from build123d import *

# Parameters (mm, degrees)
SKETCH_W     = 6
SKETCH_H     = 10
PAD_DEPTH    = 2
SKETCH001_W  = 2
SKETCH001_H  = 10
PAD001_DEPTH = 6.5
CHAMFER_SIZE = 1


with BuildPart() as part:
    # Sketch → Pad (new body)
    with BuildSketch(Plane.XY):
        Rectangle(SKETCH_W, SKETCH_H)
    extrude(amount=PAD_DEPTH)

    # Sketch001 (on Face6 of Pad) → Pad001 (join)
    with BuildSketch(Plane.XY.offset(2)):
        with Locations((-2, 0)):
            Rectangle(SKETCH001_W, SKETCH001_H)
        with Locations((2, 0)):
            Rectangle(SKETCH001_W, SKETCH001_H)
    extrude(amount=PAD001_DEPTH)

    # Chamfer
    chamfer_edges = [part.edges().sort_by_distance(p)[0] for p in [
        (-1, -5, 5.25),
        (1, -5, 5.25),
        (-1, 5, 5.25),
        (1, 5, 5.25),
    ]]
    chamfer(chamfer_edges, length=CHAMFER_SIZE)


solid = part.part
Verification items for the finished model (mm, model axes). A direction names the side the tool comes from. Round coordinates to 2 decimals unless told otherwise and drop trailing zeros. Loops run counter-clockwise (first coordinate to the right, second up) from the corner with the lowest first, then second, coordinate; pieces in that order, holes last. Notation, with made-up numbers: M 25,-26 L 77,-26 A24 ccw 77,-6 Z; hole C 27,78 d2. An arc over 180 degrees is marked long. Write each question's results on one line, items separated by ' | '.
1) Section check A-A on z = 6.5. Record the boundary of the cut face in (x, y), then the cut area to 3 significant figures.
Checks:
outline: M -3,-5 L -2,-5 L -1,-4 L -1,4 L -2,5 L -3,5 Z; M 1,-4 L 2,-5 L 3,-5 L 3,5 L 2,5 L 1,4 Z | area: 38.0 mm2
2) Section check D-D on x = -0.15. Record the boundary of the cut face in (y, z).
Checks:
outline: M -5,0 L 5,0 L 5,2 L -5,2 Z
3) Mould release check, pull along X, two halves, no side actions. Record for faces 1 (the flat face through (-3, 0, 4)), 2 (the flat face through (-2, 0, 8.5)), 3 (the flat face through (1.5, 4.5, 5.2)): released by +X, released by -X, zero draft, split by the parting line, or undercut.
Checks:
face 1: released by -X | face 2: zero draft | face 3: undercut
4) Scan lines: L1, parallel to X at y = 1, z = 6.5; L2, parallel to X at y = -4.5, z = 5.5; L3, parallel to Z at x = 0.6, y = -3.25. Record each from-to range of solid material in increasing order. Write a range as from..to.
Checks:
L1: x = -3..-1, 1..3 | L2: x = -3..-1.5, 1.5..3 | L3: z = 0..2
5) Access from +Z, -Z, +X, -X, +Y, -Y to the whole of each face (thin tool, end or side, straight path). Record for faces 4 (the flat face through (-1.5, -4.5, 5.2)), 5 (the flat face through (-1.5, 4.5, 5.2)), 6 (the flat face through (1, 0, 5)).
Checks:
face 4: +Z, -Y | face 5: +Z, +Y | face 6: +Z, +Y, -Y
6) Section check B-B on y = 4.75. Record the boundary of the cut face in (x, z).
Checks:
outline: M -3,0 L 3,0 L 3,8.5 L 1.75,8.5 L 1.75,2 L -1.75,2 L -1.75,8.5 L -3,8.5 Z
7) Section check C-C on x = -1.55. Record the boundary of the cut face in (y, z), then the cut area to 4 significant figures.
Checks:
outline: M -5,0 L 5,0 L 5,2 L 4.55,2 L 4.55,8.5 L -4.55,8.5 L -4.55,2 L -5,2 Z | area: 79.15 mm2
